CAD build for the part. Positions are in the model's coordinates, mm. A direction names the side the tool comes from. Round coordinates to 2 decimals unless told otherwise and drop trailing zeros. Loops run counter-clockwise (first coordinate to the right, second up) from the corner with the lowest first, then second, coordinate; pieces in that order, holes last. Notation, with made-up numbers: (5.25, -8.75) -> (17.25, -8.75) arc R31 ccw to (17.25, 27.25) -> close; hole circle Ø9 at (8, 70.25). An arc over 180 degrees is marked (long way). Answer as CSV lines item,"result".
```python
from build123d import *

# Parameters (mm, degrees)
F0_W     = 138.2199470003
F0_H     = 130
F1_DEPTH = 25
F2_R     = 16
F3_R     = 12
F4_DEPTH = 10
F5_W     = 3.2
F5_H     = 7.2
F6_DEPTH = 5


with BuildPart() as f1:
    # F0 (on Top) → F1 (new body)
    with BuildSketch(Plane.XY):
        with Locations((-8.8900264998, 0)):
            Rectangle(F0_W, F0_H)
    extrude(amount=F1_DEPTH)

    # F2
    f2_edges = [f1.edges().sort_by_distance(p)[0] for p in [
        (-78, -65, 12.5),
        (-78, 65, 12.5),
    ]]
    fillet(f2_edges, radius=F2_R)

    # F3
    f3_edges = [f1.edges().sort_by_distance(p)[0] for p in [
        (-0.890026, -65, 25),
    ]]
    fillet(f3_edges, radius=F3_R)

    # F4 (cut): a face of the model
    f4_faces = [f1.faces().sort_by_distance(p)[0] for p in [
        (-8.4868143179, 0, 0),
    ]]
    extrude(f4_faces, amount=-F4_DEPTH, mode=Mode.SUBTRACT)

    # F5 (on face) → F6 (cut)
    with BuildSketch(Plane.YZ.offset(60.2199470003)):
        with Locations((-43.4, 13.6)):
            Rectangle(F5_W, F5_H)
        Polygon((-1.6, 10), (0, 10), (1.6, 10), (1.6, 17.2), (0, 17.2), (-1.6, 17.2), align=None)
        with Locations((43.4, 13.6)):
            Rectangle(F5_W, F5_H)
    extrude(amount=-F6_DEPTH, mode=Mode.SUBTRACT)


solid = f1.part
```
Q1. Two-plate mould, pull along Y, no slides. Class faces 1 (the flat face through (-2, 65, 11)), 2 (the flat face through (60.22, -0.9, 17.4)), 3 (the flat face through (58, 1.6, 14)), 4 (the flat face through (58, 41.8, 14)): pulls with the +Y half, pulls with the -Y half, needs draft (parallel to the pull), parting line crosses it, or undercut.
Results:
face 1,"pulls with the +Y half"
face 2,"needs draft"
face 3,"undercut"
face 4,"undercut"
Q2. Probe L1, parallel to Y at x = -35.5, z = 19; L2, parallel to X at y = 23.5, z = 15; L3, parallel to Y at x = 49, z = 19.75. List the from-to ranges inside material, lowest first. Write a range as [from, to].
Results:
L1,"[-63.39, 63.39]"
L2,"[-77.83, 60.22]"
L3,"[-62.92, 62.92]"
Q3. Tool access for faces 5 (the flat face through (58, -43, 17.2)), 6 (the cylindrical face through (-1.75, 61.39, 21.58)): list every direction of +Z, -Z, +X, -X, +Y, -Y with a clear straight run to the whole face (end or side of a thin tool).
Results:
face 5,"-Z, +X"
face 6,"+Z, +X, -X, +Y"
Q4. Slice it at A-A, the plane x = -58.5. Give the cut face in (y, z).
Results:
outline,"(-65, 10) -> (65, 10) -> (65, 13) arc R12 ccw to (53, 25) -> (-53, 25) arc R12 ccw to (-65, 13) -> close"
Q5. Drop flat-ended pins along their axis: pin 1 Ø3.5 at (x, y) = (57, 43) entering from -Z; pin 2 Ø1.6 at (x, y) = (59, -0.5) entering from -Z; pin 3 Ø1.6 at (y, z) = (0, 13) entering from +X; pin 4 Ø8 at (x, z) = (-29, 20.5) entering from -Y. Give the stop position or say it passes through.
Results:
pin 1,"z = 10"
pin 2,"z = 17.2"
pin 3,"x = 55.22"
pin 4,"y = -64.48"
